Part model, mm, in its own coordinate system. Face numbers are marked on the shaded views. A direction names the side the tool comes from. Round coordinates to 2 decimals unless told otherwise and drop trailing zeros. Loops run counter-clockwise (first coordinate to the right, second up) from the corner with the lowest first, then second, coordinate; pieces in that order, holes last. Notation, with made-up numbers: (-4.75, 31) -> (43.25, 31) arc R25 ccw to (43.25, 55) -> close; hole circle Ø1 at (77.5, -29.75). An arc over 180 degrees is marked (long way). Use a Markdown table: item, result. Add a question column.
Item 1: Cut at B-B, the plane z = 8.25. List the corners of the cut face in (x, y).
Item 2: Cut at A-A, the plane x = 59.25. List the corners of the cut face in (y, z).
Item 3: Which spindle directions (+Z, -Z, +X, -X, +Y, -Y) get a long thin tool onto all of the face, cutting with end or side? Do the marked faces 1, 2 and 3. Say none if no direction does.
Item 4: Flat gauge pins, fed straight in: pin 1 (3.5 mm diameter, centred on x = 66.74, z = 16, fed in from -Y); pin 2 (3 mm diameter, centred on y = -6.5, z = 16, fed in from +X); pin 3 (1.5 mm diameter, centred on y = -25.5, z = 10, fed in from -X); pin 4 (4 mm diameter, centred on y = -15.5, z = 20, fed in from -X). Where does each tip first touch, or does it go through?
Item 5: Two-plate mould, pull along Z, no slides. Class the marked faces 4, 5 and 6: pulls with the +Z half, pulls with the -Z half, needs draft (parallel to the pull), parting line crosses it, or undercut.
Item 6: Probe line 1 (Z direction, x = 59.75, y = -22); line 2 (X direction, y = -39, z = 9); line 3 (Z direction, x = 66, y = -9). List the from-to ranges inside material, lowest first. Write a range as [from, to].
Item 7: Cut at C-C, the plane y = -4. State how many separate pieces and enclosed holes the cut face has, plus the area to 3 significant figures.
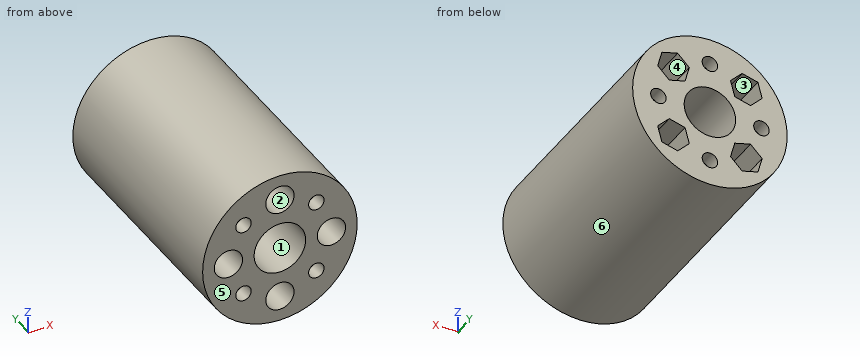
```python
from build123d import *

# Parameters (mm, degrees)
SKETCH_1_R               = 15
SKETCH_1_R_2             = 5
EXTRUDE_4_DEPTH          = 3
SKETCH_1_R_3             = 3.5
SKETCH_1_R_4             = 2.1
EXTRUDE_4_2_DEPTH        = 3
EXTRUDE_5_DEPTH          = 3
PATTERN_CIRCULAR_2_COUNT = 4
SKETCH_6_R               = 3.5
SKETCH_6_R_2             = 2.1
EXTRUDE_6_DEPTH          = 3
PATTERN_CIRCULAR_3_COUNT = 4
SKETCH_7_R               = 15
SKETCH_7_R_2             = 5
EXTRUDE_7_DEPTH          = 46
CUT_EXTRUDE_1_DEPTH      = 46
PATTERN_CIRCULAR_4_COUNT = 4
SKETCH_11_R              = 1.5
CUT_EXTRUDE_2_DEPTH      = 3
PATTERN_CIRCULAR_5_COUNT = 4
EXTRUDE_8_DEPTH          = 3
EXTRUDE_9_DEPTH          = 3
EXTRUDE_10_DEPTH         = 3
EXTRUDE_11_DEPTH         = 3
EXTRUDE_13_DEPTH         = 3
EXTRUDE_14_DEPTH         = 3
CUT_EXTRUDE_3_DEPTH      = 2.5
SKETCH_19_R              = 1.5
CUT_EXTRUDE_4_DEPTH      = 2.5
SKETCH_20_R              = 1.5
CUT_EXTRUDE_5_DEPTH      = 2.5
SKETCH_21_R              = 15
SKETCH_21_R_2            = 5
EXTRUDE_15_DEPTH         = 3
SKETCH_22_R              = 1.5
CUT_EXTRUDE_6_DEPTH      = 3
PATTERN_CIRCULAR_6_COUNT = 4
EXTRUDE_16_DEPTH         = 3
CUT_EXTRUDE_7_DEPTH      = 3
SKETCH_25_R              = 15
SKETCH_25_R_2            = 5
EXTRUDE_17_DEPTH         = 43
SKETCH_27_R              = 1.5
CUT_EXTRUDE_8_DEPTH      = 46
SKETCH_28_R              = 2.75
CUT_EXTRUDE_9_DEPTH      = 43
SKETCH_29_R              = 1.5
CUT_EXTRUDE_10_DEPTH     = 46
PATTERN_CIRCULAR_7_COUNT = 4
CUT_EXTRUDE_11_DEPTH     = 43
PATTERN_CIRCULAR_8_COUNT = 4
SKETCH_31_R              = 43.855676254
CUT_EXTRUDE_12_DEPTH     = 100


with BuildPart() as part:
    # Sketch 1 → Extrude 4 (new body)
    with BuildSketch(Plane(origin=(0, 0, 0), x_dir=(1, 0, 0), z_dir=(0, 1, 0))):
        with Locations((-5.372895461, -8.931727747)):
            Circle(SKETCH_1_R)
        with Locations((-5.372895461, -8.931727747)):
            Circle(SKETCH_1_R_2, mode=Mode.SUBTRACT)
    extrude(amount=EXTRUDE_4_DEPTH)



with BuildPart() as body_2:
    # Sketch 1 → Extrude 4 2 (new body)
    with BuildSketch(Plane(origin=(0, 0, 0), x_dir=(1, 0, 0), z_dir=(0, 1, 0))):
        with Locations((-22.372895461, 8.068272253)):
            Circle(SKETCH_1_R_3)
        with Locations((-22.372895461, 8.068272253)):
            Circle(SKETCH_1_R_4, mode=Mode.SUBTRACT)
    extrude(amount=EXTRUDE_4_2_DEPTH)


with BuildPart() as part_1:
    add(part.part)

    add(body_2.part)  # Extrude 5 merges body 2
    # Sketch 5 → Extrude 5 (add)
    with BuildSketch(Plane(origin=(0, 0, 0), x_dir=(1, 0, 0), z_dir=(0, 1, 0))):
        Polygon((-22.372895461, 4.568272253), (-10.372895461, -8.931727747), (-10.372895461, -3.931727747), (-5.372895461, -3.931727747), (-18.872895461, 8.068272253), align=None)
    extrude_5 = extrude(amount=EXTRUDE_5_DEPTH)

    # Pattern Circular 2: Extrude 5 ×4 about axis
    pattern_circular_2_axis = Axis((-5.372895461, 0, 8.931727747), (0, 1, 0))
    for i in range(1, PATTERN_CIRCULAR_2_COUNT):
        add(extrude_5.rotate(pattern_circular_2_axis, i * 360 / PATTERN_CIRCULAR_2_COUNT))

    # Sketch 6 → Extrude 6 (add)
    with BuildSketch(Plane(origin=(0, 3, 0), x_dir=(1, 0, 0), z_dir=(0, 1, 0))):
        with Locations((11.627104539, 8.068272253)):
            Circle(SKETCH_6_R)
        with Locations((11.627104539, 8.068272253)):
            Circle(SKETCH_6_R_2, mode=Mode.SUBTRACT)
    extrude_6 = extrude(amount=-EXTRUDE_6_DEPTH)

    # Pattern Circular 3: Extrude 6 ×4 about axis
    pattern_circular_3_axis = Axis((-5.372895461, 0, 8.931727747), (0, 1, 0))
    for i in range(1, PATTERN_CIRCULAR_3_COUNT):
        add(extrude_6.rotate(pattern_circular_3_axis, i * 360 / PATTERN_CIRCULAR_3_COUNT))

    # Sketch 7 → Extrude 7 (add)
    with BuildSketch(Plane.XZ):
        with Locations((-5.372895461, 8.931727747)):
            Circle(SKETCH_7_R)
        with Locations((-5.372895461, 8.931727747)):
            Circle(SKETCH_7_R_2, mode=Mode.SUBTRACT)
    extrude(amount=EXTRUDE_7_DEPTH)

    # Sketch 9 → Cut-Extrude 1 (cut)
    with BuildSketch(Plane(origin=(0, 3, 0), x_dir=(1, 0, 0), z_dir=(0, 1, 0))):
        Polygon((0.876311502, -19.070022006), (-1.369054096, -16.824656408), (-0.547193246, -13.757429961), (2.520033201, -12.935569112), (4.765398798, -15.180934709), (3.943537949, -18.248161156), align=None)
    cut_extrude_1 = extrude(amount=-CUT_EXTRUDE_1_DEPTH, mode=Mode.SUBTRACT)

    # Pattern Circular 4: Cut-Extrude 1 ×4 about axis
    pattern_circular_4_axis = Axis((-5.372895461, 0, 8.931727747), (0, 1, 0))
    for i in range(1, PATTERN_CIRCULAR_4_COUNT):
        add(cut_extrude_1.rotate(pattern_circular_4_axis, i * 360 / PATTERN_CIRCULAR_4_COUNT), mode=Mode.SUBTRACT)

    # Sketch 11 → Cut-Extrude 2 (cut)
    with BuildSketch(Plane(origin=(0, -43, 0), x_dir=(1, 0, 0), z_dir=(0, 1, 0))):
        with Locations((1.698172351, -1.860659935)):
            Circle(SKETCH_11_R)
    cut_extrude_2 = extrude(amount=-CUT_EXTRUDE_2_DEPTH, mode=Mode.SUBTRACT)

    # Pattern Circular 5: Cut-Extrude 2 ×4 about axis
    pattern_circular_5_axis = Axis((-5.372895461, 0, 8.931727747), (0, 1, 0))
    for i in range(1, PATTERN_CIRCULAR_5_COUNT):
        add(cut_extrude_2.rotate(pattern_circular_5_axis, i * 360 / PATTERN_CIRCULAR_5_COUNT), mode=Mode.SUBTRACT)

    # Sketch 12 → Extrude 8 (add)
    with BuildSketch(Plane(origin=(0, 3, 0), x_dir=(1, 0, 0), z_dir=(0, 1, 0))):
        Polygon((15.127104539, 8.068272253), (15.127104539, -25.931727747), (11.627104539, -22.431727747), (11.627104539, 4.568272253), align=None)
    extrude(amount=-EXTRUDE_8_DEPTH)

    # Sketch 13 → Extrude 9 (add)
    with BuildSketch(Plane(origin=(0, 3, 0), x_dir=(1, 0, 0), z_dir=(0, 1, 0))):
        Polygon((11.627104539, 11.568272253), (-22.372895461, 11.568272253), (-18.872895461, 8.068272253), (8.127104539, 8.068272253), align=None)
    extrude(amount=-EXTRUDE_9_DEPTH)

    # Sketch 14 → Extrude 10 (add)
    with BuildSketch(Plane(origin=(0, 3, 0), x_dir=(1, 0, 0), z_dir=(0, 1, 0))):
        Polygon((-25.872895461, 8.068272253), (-25.872895461, -25.931727747), (-22.372895461, -22.431727747), (-22.372895461, 4.568272253), align=None)
    extrude(amount=-EXTRUDE_10_DEPTH)

    # Sketch 15 → Extrude 11 (add)
    with BuildSketch(Plane(origin=(0, 3, 0), x_dir=(1, 0, 0), z_dir=(0, 1, 0))):
        Polygon((-22.372895461, -29.431727747), (11.627104539, -29.431727747), (8.127104539, -25.931727747), (-18.872895461, -25.931727747), align=None)
    extrude(amount=-EXTRUDE_11_DEPTH)

    # Sketch 16 → Extrude 13 (add)
    with BuildSketch(Plane.XZ):
        Polygon((-10.747895461, -4.193272253), (0.002104539, -4.193272253), (5.163560245, -8.068272253), (4.99115505, -11.568272253), (0.002104539, -14.943272253), (-10.747895461, -14.943272253), (-15.736945971, -11.568272253), (-15.909351166, -8.068272253), align=None)
        Polygon((-7.57246898, -9.568272253), (-9.16018222, -6.818272253), (-12.335608701, -6.818272253), (-13.923321941, -9.568272253), (-12.335608701, -12.318272253), (-9.16018222, -12.318272253), align=None, mode=Mode.SUBTRACT)
        Polygon((3.17753102, -9.568272253), (1.58981778, -6.818272253), (-1.585608701, -6.818272253), (-3.173321941, -9.568272253), (-1.585608701, -12.318272253), (1.58981778, -12.318272253), align=None, mode=Mode.SUBTRACT)
    extrude(amount=-EXTRUDE_13_DEPTH)

    # Sketch 18 → Extrude 14 (add)
    with BuildSketch(Plane.XZ):
        Polygon((-7.57246898, -9.568272253), (-9.16018222, -6.818272253), (-12.335608701, -6.818272253), (-13.923321941, -9.568272253), (-12.335608701, -12.318272253), (-9.16018222, -12.318272253), align=None)
        Polygon((3.17753102, -9.568272253), (1.58981778, -6.818272253), (-1.585608701, -6.818272253), (-3.173321941, -9.568272253), (-1.585608701, -12.318272253), (1.58981778, -12.318272253), align=None)
    extrude(amount=-EXTRUDE_14_DEPTH)

    # Sketch 17 → Cut-Extrude 3 (cut)
    with BuildSketch(Plane.XZ):
        Polygon((-7.57246898, -9.568272253), (-9.16018222, -6.818272253), (-12.335608701, -6.818272253), (-13.923321941, -9.568272253), (-12.335608701, -12.318272253), (-9.16018222, -12.318272253), align=None)
        Polygon((3.17753102, -9.568272253), (1.58981778, -6.818272253), (-1.585608701, -6.818272253), (-3.173321941, -9.568272253), (-1.585608701, -12.318272253), (1.58981778, -12.318272253), align=None)
    extrude(amount=-CUT_EXTRUDE_3_DEPTH, mode=Mode.SUBTRACT)

    # Sketch 19 → Cut-Extrude 4 (cut)
    with BuildSketch(Plane.XZ.offset(-2.5)):
        with Locations((0.002104539, -9.568272253)):
            Circle(SKETCH_19_R)
    extrude(amount=-CUT_EXTRUDE_4_DEPTH, mode=Mode.SUBTRACT)

    # Sketch 20 → Cut-Extrude 5 (cut)
    with BuildSketch(Plane.XZ.offset(-2.5)):
        with Locations((-10.747895461, -9.568272253)):
            Circle(SKETCH_20_R)
    extrude(amount=-CUT_EXTRUDE_5_DEPTH, mode=Mode.SUBTRACT)

    # Sketch 8 → Extrude 16 (add)
    with BuildSketch(Plane.XZ.offset(46)):
        Polygon((3.943537949, 18.248161156), (0.876311502, 19.070022006), (-1.369054096, 16.824656408), (-0.547193246, 13.757429961), (2.520033201, 12.935569112), (4.765398798, 15.180934709), align=None)
    extrude(amount=EXTRUDE_16_DEPTH)

    # Sketch 24 → Cut-Extrude 7 (cut)
    with BuildSketch(Plane.XZ.offset(49)):
        Polygon((4.765398798, 15.180934709), (3.943537949, 18.248161156), (0.876311502, 19.070022006), (-1.369054096, 16.824656408), (-0.547193246, 13.757429961), (2.520033201, 12.935569112), align=None)
    extrude(amount=-CUT_EXTRUDE_7_DEPTH, mode=Mode.SUBTRACT)

    # Sketch 31 → Cut-Extrude 12 (cut)
    with BuildSketch(Plane(origin=(0, 3, 0), x_dir=(1, 0, 0), z_dir=(0, 1, 0))):
        with Locations((-6.865297473, -8.372369535)):
            Circle(SKETCH_31_R)
    extrude(amount=-CUT_EXTRUDE_12_DEPTH, mode=Mode.SUBTRACT)


with BuildPart() as body_2_2:
    # Sketch 21 → Extrude 15 (new body)
    with BuildSketch(Plane(origin=(0, 0, 0), x_dir=(1, 0, 0), z_dir=(0, 1, 0))):
        with Locations((59.665545214, -8.931727747)):
            Circle(SKETCH_21_R)
        with Locations((59.665545214, -8.931727747)):
            Circle(SKETCH_21_R_2, mode=Mode.SUBTRACT)
    extrude(amount=EXTRUDE_15_DEPTH)

    # Sketch 22 → Cut-Extrude 6 (cut)
    with BuildSketch(Plane.XZ):
        with Locations((59.665545214, 18.931727747)):
            Circle(SKETCH_22_R)
    cut_extrude_6 = extrude(amount=-CUT_EXTRUDE_6_DEPTH, mode=Mode.SUBTRACT)

    # Pattern Circular 6: Cut-Extrude 6 ×4 about axis
    pattern_circular_6_axis = Axis((59.665545214, 0, 8.931727747), (0, 1, 0))
    for i in range(1, PATTERN_CIRCULAR_6_COUNT):
        add(cut_extrude_6.rotate(pattern_circular_6_axis, i * 360 / PATTERN_CIRCULAR_6_COUNT), mode=Mode.SUBTRACT)

    # Sketch 25 → Extrude 17 (add)
    with BuildSketch(Plane.XZ):
        with Locations((59.665545214, 8.931727747)):
            Circle(SKETCH_25_R)
        with Locations((59.665545214, 8.931727747)):
            Circle(SKETCH_25_R_2, mode=Mode.SUBTRACT)
    extrude(amount=EXTRUDE_17_DEPTH)

    # Sketch 27 → Cut-Extrude 8 (cut)
    with BuildSketch(Plane(origin=(0, 3, 0), x_dir=(1, 0, 0), z_dir=(0, 1, 0))):
        with Locations((59.665545214, 1.068272253)):
            Circle(SKETCH_27_R)
        with Locations((69.665545214, -8.931727747)):
            Circle(SKETCH_27_R)
        with Locations((59.665545214, -18.931727747)):
            Circle(SKETCH_27_R)
        with Locations((49.665545214, -8.931727747)):
            Circle(SKETCH_27_R)
    extrude(amount=-CUT_EXTRUDE_8_DEPTH, mode=Mode.SUBTRACT)

    # Sketch 28 → Cut-Extrude 9 (cut)
    with BuildSketch(Plane.XZ.offset(43)):
        with Locations((59.665545214, 18.931727747)):
            Circle(SKETCH_28_R)
        with Locations((49.665545214, 8.931727747)):
            Circle(SKETCH_28_R)
        with Locations((59.665545214, -1.068272253)):
            Circle(SKETCH_28_R)
        with Locations((69.665545214, 8.931727747)):
            Circle(SKETCH_28_R)
    extrude(amount=-CUT_EXTRUDE_9_DEPTH, mode=Mode.SUBTRACT)

    # Sketch 29 → Cut-Extrude 10 (cut)
    with BuildSketch(Plane(origin=(0, 3, 0), x_dir=(1, 0, 0), z_dir=(0, 1, 0))):
        with Locations((66.736613026, -1.860659935)):
            Circle(SKETCH_29_R)
    cut_extrude_10 = extrude(amount=-CUT_EXTRUDE_10_DEPTH, mode=Mode.SUBTRACT)

    # Pattern Circular 7: Cut-Extrude 10 ×4 about axis
    pattern_circular_7_axis = Axis((59.665545214, 0, 8.931727747), (0, 1, 0))
    for i in range(1, PATTERN_CIRCULAR_7_COUNT):
        add(cut_extrude_10.rotate(pattern_circular_7_axis, i * 360 / PATTERN_CIRCULAR_7_COUNT), mode=Mode.SUBTRACT)

    # Sketch 30 → Cut-Extrude 11 (cut)
    with BuildSketch(Plane(origin=(0, 3, 0), x_dir=(1, 0, 0), z_dir=(0, 1, 0))):
        Polygon((64.491247429, -4.106025533), (67.558473876, -4.927886382), (69.803839473, -2.682520785), (68.981978624, 0.384705662), (65.914752177, 1.206566512), (63.669386579, -1.038799086), align=None)
    cut_extrude_11 = extrude(amount=-CUT_EXTRUDE_11_DEPTH, mode=Mode.SUBTRACT)

    # Pattern Circular 8: Cut-Extrude 11 ×4 about axis
    pattern_circular_8_axis = Axis((59.665545214, 0, 8.931727747), (0, 1, 0))
    for i in range(1, PATTERN_CIRCULAR_8_COUNT):
        add(cut_extrude_11.rotate(pattern_circular_8_axis, i * 360 / PATTERN_CIRCULAR_8_COUNT), mode=Mode.SUBTRACT)


solid = body_2_2.part
```
A:
| question | item | result |
|---|---|---|
| 1 | outline | (44.68, -43) -> (47, -43) -> (47, 0) -> (48.33, 0) -> (48.33, 3) -> (44.68, 3) -> close; (51, 0) -> (52.33, 0) -> (52.33, -43) -> (54.71, -43) -> (54.71, 3) -> (51, 3) -> close; (64.62, -43) -> (67, -43) -> (67, 0) -> (68.33, 0) -> (68.33, 3) -> (64.62, 3) -> close; (71, 0) -> (72.33, 0) -> (72.33, -43) -> (74.65, -43) -> (74.65, 3) -> (71, 3) -> close |
| 2 | outline | (-43, -6.06) -> (3, -6.06) -> (3, -2.51) -> (0, -2.51) -> (0, -3.79) -> (-43, -3.79) -> close; (-43, 1.65) -> (0, 1.65) -> (0, 0.37) -> (3, 0.37) -> (3, 3.95) -> (-43, 3.95) -> close; (-43, 13.91) -> (3, 13.91) -> (3, 17.49) -> (0, 17.49) -> (0, 16.21) -> (-43, 16.21) -> close; (-43, 21.65) -> (0, 21.65) -> (0, 20.37) -> (3, 20.37) -> (3, 23.93) -> (-43, 23.93) -> close |
| 3 | face 1 | +Y, -Y |
| 3 | face 2 | -Y |
| 3 | face 3 | +Y |
| 4 | pin 1 | stops at y = -43 |
| 4 | pin 2 | stops at x = 73.59 |
| 4 | pin 3 | stops at x = 44.67 |
| 4 | pin 4 | stops at x = 47.72 |
| 5 | face 4 | undercut |
| 5 | face 5 | needs draft |
| 5 | face 6 | parting line crosses it |
| 6 | line 1 | z = [-6.07, -3.82], [1.68, 3.93], [13.93, 16.18], [21.68, 23.93] |
| 6 | line 2 | x = [44.67, 46.92], [52.41, 54.67], [64.67, 66.92], [72.41, 74.67] |
| 6 | line 3 | z = [-4.67, -1.18], [4.51, 13.35], [19.05, 22.53] |
| 7 | separate pieces | 1 |
| 7 | enclosed holes | 9 |
| 7 | area | 428 mm^2 |
